Geometry check sheet. Reference: the model listing, model coordinates, mm. A direction names the side the tool comes from. Coordinates: 2 decimals unless noted, no trailing zeros. Write each loop counter-clockwise with the first axis right and the second up, starting at its lowest first coordinate (ties: lowest second). Pieces come first, ordered by that corner, then holes. Notation, with made-up numbers: (20, 49) -> (71, 49) arc R17 cw to (71, 75) -> close; hole circle Ø4 at (51.5, 0.25). An arc over 180 degrees is marked (long way). Use a Markdown table: item, result.
```python
from build123d import *

# Parameters (mm, degrees)
F0_W     = 16.1465890706
F0_H     = 50
F1_DEPTH = 100
F0_W_2   = 82.4685227126
F2_DEPTH = 8.5
F3_SIZE  = 15
F4_W     = 50
F4_H     = 137.2287848778
F5_DEPTH = 28
F4_H_2   = 21.2132034356
F4_H_3   = 116.0155814422
F6_DEPTH = 2
F0_H_2   = 30.8768022805
F0_H_3   = 19.9685309082
F7_DEPTH = 25


with BuildPart() as f1:
    # F0 (on Top) → F1 (new body)
    with BuildSketch(Plane.XY):
        with Locations((66.7468514293, 8.8534165174)):
            Rectangle(F0_W, F0_H)
    extrude(amount=F1_DEPTH)

    # F0 (on Top) → F2 (join)
    with BuildSketch(Plane.XY):
        with Locations((17.4392955378, 8.8534165174)):
            Rectangle(F0_W_2, F0_H)
    extrude(amount=F2_DEPTH)

    # F3
    f3_edges = [f1.edges().sort_by_distance(p)[0] for p in [
        (58.673557, 8.853417, 100),
    ]]
    chamfer(f3_edges, length=F3_SIZE)

    # F4 (on face) → F5 (cut)
    with BuildSketch(Plane(origin=(-13.163221553, 0, 13.163221553), x_dir=(0, -1, 0), z_dir=(-0.7071067812, 0, 0.7071067812))):
        with Locations((-8.8534165174, 54.1913573537)):
            Rectangle(F4_W, F4_H)
    extrude(amount=F5_DEPTH, mode=Mode.SUBTRACT)

    # F4 (on face) → F6 (join)
    with BuildSketch(Plane(origin=(-13.163221553, 0, 13.163221553), x_dir=(0, -1, 0), z_dir=(-0.7071067812, 0, 0.7071067812))):
        with Locations((-8.8534165174, 112.1991480748)):
            Rectangle(F4_W, F4_H_2)
        with Locations((-8.8534165174, 43.5847556359)):
            Rectangle(F4_W, F4_H_3)
    extrude(amount=F6_DEPTH)

    # F0 (on Top) → F7 (join)
    with BuildSketch(Plane.XY):
        with Locations((66.7468514293, -31.5849846229)):
            Rectangle(F0_W, F0_H_2)
        with Locations((66.7468514293, 43.8376819715)):
            Rectangle(F0_W, F0_H_3)
    extrude(amount=F7_DEPTH)


solid = f1.part
```
Item 1: Section check C-C on z = 13. Record the boundary of the cut face in (x, y).
Answer block:
| item | result |
|---|---|
| outline | (-16.15, -16.15) -> (-13.33, -16.15) -> (-13.33, 33.85) -> (-16.15, 33.85) -> close; (58.67, -47.02) -> (74.82, -47.02) -> (74.82, 53.82) -> (58.67, 53.82) -> close |
Item 2: Section check A-A on y = 11.5. Record the boundary of the cut face in (x, z), then the cut area to 3 significant figures.
Answer block:
| item | result |
|---|---|
| outline | (-24.78, 4.38) -> (-23.79, 3.4) -> (-23.79, 0) -> (74.82, 0) -> (74.82, 100) -> (73.67, 100) -> (72.26, 101.41) -> close; hole (-17.83, 8.5) -> (58.67, 8.5) -> (58.67, 85) -> close |
| area | 2,460 mm^2 |
Item 3: Section check B-B on x = 6. Record the boundary of the cut face in (y, z).
Answer block:
| item | result |
|---|---|
| outline | (-16.15, 0) -> (33.85, 0) -> (33.85, 8.5) -> (-16.15, 8.5) -> close; (-16.15, 32.33) -> (33.85, 32.33) -> (33.85, 35.15) -> (-16.15, 35.15) -> close |
Item 4: Tool access check on faces 5 (the flat face through (61, 33.853, 37)), 6 (the flat face through (-23.795, 9, 2)), 7 (the flat face through (67, 44, 25)), 8 (the flat face through (59, -16.147, 38)). Record the directions out of +Z, -Z, +X, -X, +Y, -Y that give a thin tool (end or side, any length) a straight path to the whole face; none if there is none.
Answer block:
| item | result |
|---|---|
| face 5 | +Z, -X, +Y |
| face 6 | -Z, -X, +Y, -Y |
| face 7 | +Z, +X, -X, +Y |
| face 8 | +Z, -X, -Y |
Item 5: Thickness scan on L1, parallel to Y at x = 59, z = 26; L2, parallel to Z at x = 32.5, y = 26; L3, parallel to Z at x = 47.5, y = 32.5. Record the ranges inside material, lowest first. Write a range as [from, to].
Answer block:
| item | result |
|---|---|
| L1 | y = [-16.15, 33.85] |
| L2 | z = [0, 8.5], [58.83, 61.65] |
| L3 | z = [0, 8.5], [73.83, 76.65] |
Item 6: Mould release check, pull along Z, two halves, no side actions. Record for faces 1 (the flat face through (67, -31, 25)), 2 (the flat face through (20, 9, 8.5)), 3 (the flat face through (74.82, 3, 38)), 4 (the flat face through (20.959, 9.203, 47.286)): +Z half, -Z half, draft (parallel to the pull), parting line (faces both ways), or undercut.
Answer block:
| item | result |
|---|---|
| face 1 | +Z half |
| face 2 | undercut |
| face 3 | draft |
| face 4 | undercut |
Item 7: Depth check by flat-ended pin: P1, Ø2, axis at x = 5.5, z = 34.5, coming from the +Y side; P2, Ø18, axis at x = 67, y = -26.5, coming from the +Z side; P3, Ø3.5, axis at y = 21.5, z = 1, coming from the -X side. Enter the tip coordinate at first touch or a pass-through.
Answer block:
| item | result |
|---|---|
| P1 | stops at y = 33.85 |
| P2 | stops at z = 25 |
| P3 | stops at x = -23.79 |
